Verification items for the finished model (mm, model axes). Round coordinates to 2 decimals unless told otherwise and drop trailing zeros. Write each loop counter-clockwise with the first axis right and the second up, starting at its lowest first coordinate (ties: lowest second). Pieces come first, ordered by that corner, then holes. Notation, with made-up numbers: (51.5, 81.25) - (101.5, 81.25) arc R13 ccw to (101.5, 92.25) - close; hole circle Ø2 at (18.25, 5). An arc over 180 degrees is marked (long way). Answer as a JSON object with one key per item and string values.
```python
from build123d import *

# Parameters (mm, degrees)
F0_W     = 25.4605272785
F0_H     = 12.7302636392
F1_DEPTH = 51
F2_R     = 3.6756964622
F3_DEPTH = 25
F4_R     = 3.3400093655
F5_DEPTH = 25
F6_R     = 5.3474190326
F7_DEPTH = 25


# Not quite as in the source:
# - a feature names something its author has since deleted; it is built from what else it names


with BuildPart() as f1:
    # F0 (on Top) → F1 (new body)
    with BuildSketch(Plane.XY):
        with Locations((1.0361843742, 1.1842104141)):
            Rectangle(F0_W, F0_H)
    extrude(amount=F1_DEPTH)

    # F2 (on face) → F3 (cut)
    with BuildSketch(Plane(origin=(0, 7.5493422337, 0), x_dir=(-1, 0, 0), z_dir=(0, 1, 0))):
        with Locations((-6.8494305015, 44.5928275585)):
            Circle(F2_R)
    extrude(amount=-F3_DEPTH, mode=Mode.SUBTRACT)

    # F4 (on face) → F5 (cut)
    with BuildSketch(Plane(origin=(0, 7.5493422337, 0), x_dir=(-1, 0, 0), z_dir=(0, 1, 0))):
        with Locations((4.7804336064, 44.4043427706)):
            Circle(F4_R)
    extrude(amount=-F5_DEPTH, mode=Mode.SUBTRACT)

    # F6 (on face) → F7 (cut)
    with BuildSketch(Plane.XZ.offset(5.1809214056)):
        with Locations((0, 11.1019741744)):
            Circle(F6_R)
    extrude(amount=-F7_DEPTH, mode=Mode.SUBTRACT)


solid = f1.part
```
Q1. Section check A-A, the plane x = 0. Record the cut outline in (y, z).
Geometry check:
{"outline": "(-5.18, 0) - (7.55, 0) - (7.55, 5.75) - (-5.18, 5.75) - close; (-5.18, 16.45) - (7.55, 16.45) - (7.55, 51) - (-5.18, 51) - close"}
Q2. Section check C-C, the plane y = -2. Record the cut outline in (x, z).
Geometry check:
{"outline": "(-11.69, 0) - (13.77, 0) - (13.77, 51) - (-11.69, 51) - close; hole circle Ø6.68 at (-4.78, 44.4); hole circle Ø10.69 at (0, 11.1); hole circle Ø7.35 at (6.85, 44.59)"}
Q3. Section check D-D, the plane z = 42. Record the cut outline in (x, y).
Geometry check:
{"outline": "(-11.69, -5.18) - (-7.1, -5.18) - (-7.1, 7.55) - (-11.69, 7.55) - close; (-2.46, -5.18) - (4.24, -5.18) - (4.24, 7.55) - (-2.46, 7.55) - close; (9.45, -5.18) - (13.77, -5.18) - (13.77, 7.55) - (9.45, 7.55) - close"}
Q4. Release check for a two-part mould opening along X. For faces 1 (the flat face through (13.766, 1, 25)), 2 (the flat face through (1, 1, 51)), 3 (the cylindrical face through (7.646, 1.273, 41.005)) record: released by +X, released by -X, zero draft, split by the parting line, or undercut.
Geometry check:
{"face 1": "released by +X", "face 2": "zero draft", "face 3": "undercut"}
Q5. Section check B-B, the plane z = 8.5. Record the cut outline in (x, y).
Geometry check:
{"outline": "(-11.69, -5.18) - (-4.67, -5.18) - (-4.67, 7.55) - (-11.69, 7.55) - close; (4.67, -5.18) - (13.77, -5.18) - (13.77, 7.55) - (4.67, 7.55) - close"}
Q6. Material ranges on line 1 along Z through (x, y) = (0, 2.75); line 2 along X through (y, z) = (-3.5, 43); line 3 along Z through (x, y) = (-4.5, 2.5), recorded low to high. Write a range as [from, to].
Geometry check:
{"line 1": "z = [0, 5.75], [16.45, 51]", "line 2": "x = [-11.69, -7.81], [-1.75, 3.54], [10.16, 13.77]", "line 3": "z = [0, 8.21], [13.99, 41.08], [47.73, 51]"}
